from build123d import *

# Parameters (mm, degrees)
BOSS_EXTRUDE1_DEPTH      = 19.05
BOSS_EXTRUDE1_DEPTH_BACK = 54.61
SKETCH2_R                = 3.2512
CUT_EXTRUDE1_DEPTH       = 9.525
FILLET1_R                = 1.27


with BuildPart() as part:
    # Sketch1 → Boss-Extrude1 (new, two sides: drawn at the far end of the back side and taken through both)
    with BuildSketch(Plane(origin=(0, 0, 0), x_dir=(1, 0, 0), z_dir=(0, 1, 0)).offset(-BOSS_EXTRUDE1_DEPTH_BACK)):
        with BuildLine():
            Line((6.1595, -12.990051451), (6.1595, -27.747157521))
            ThreePointArc((6.1595, -27.747157521), (0, -28.4226), (-6.1595, -27.747157521))
            Line((-6.1595, -27.747157521), (-6.1595, -12.990051451))
            ThreePointArc((-6.1595, -12.990051451), (0, -14.3764), (6.1595, -12.990051451))
        make_face()
    extrude(amount=BOSS_EXTRUDE1_DEPTH + BOSS_EXTRUDE1_DEPTH_BACK)

    # Sketch2 → Cut-Extrude1 (cut, symmetric)
    with BuildSketch(Plane(origin=(0, 0, 0), x_dir=(0, 0, -1), z_dir=(1, 0, 0))):
        with Locations((-20.6375, 12.7)):
            Circle(SKETCH2_R)
        with Locations((-20.6375, -48.26)):
            Circle(SKETCH2_R)
    extrude(amount=CUT_EXTRUDE1_DEPTH, both=True, mode=Mode.SUBTRACT)

    # Fillet1
    fillet1_edges = [part.edges().sort_by_distance(p)[0] for p in [
        (0, -54.61, 28.4226),
        (0, 19.05, 14.3764),
        (-6.1595, 19.05, 20.368604486),
        (6.1595, -54.61, 20.368604486),
        (0, 19.05, 28.4226),
        (6.1595, 19.05, 20.368604486),
        (0, -54.61, 14.3764),
        (-6.1595, -54.61, 20.368604486),
        (6.1595, -17.78, 12.990051451),
        (6.1595, -17.78, 27.747157521),
        (-6.1595, -17.78, 27.747157521),
        (-6.1595, -17.78, 12.990051451),
    ]]
    fillet(fillet1_edges, radius=FILLET1_R)


solid = part.part
Read the model definition and answer for the solid it produces. Units are mm, in the model's axes. Coordinates: 2 decimals unless noted, no trailing zeros. Order: outer loops, then holes, each group sorted by start corner. A loop starts at its lowest first (then second) coordinate and runs counter-clockwise, first axis right, second up. Notation, with made-up numbers: (17, 74) - (29, 74) arc R20 ccw to (29, 98) - close; hole circle Ø10 at (-26.5, 53). An arc over 180 degrees is marked (long way). Use one line per item in the form item = value.
(1) Given pin 1 Ø4 at (x, y) = (0.5, -25) entering from -Z; pin 2 Ø6 at (x, y) = (3.5, -17) entering from +Z; pin 3 Ø1.5 at (x, y) = (3.5, -14.5) entering from -Z, each flat-ended and moving along its own axis, determine where each tip first touches the part or whether it passes through.
Computed values:
pin_1 = 14.16
pin_2 = 28.42
pin_3 = 13.73
(2) Section D-D, the plane z = 18.5 is taken. Give the vertices of the cut face in (x, y).
Computed values:
outline = (-6.16, -53.34) arc R1.27 ccw to (-4.89, -54.61) - (4.89, -54.61) arc R1.27 ccw to (6.16, -53.34) - (6.16, -50.71) - (-6.16, -50.71) - close; (-6.16, -45.81) - (6.16, -45.81) - (6.16, 10.25) - (-6.16, 10.25) - close; (-6.16, 15.15) - (6.16, 15.15) - (6.16, 17.78) arc R1.27 ccw to (4.89, 19.05) - (-4.89, 19.05) arc R1.27 ccw to (-6.16, 17.78) - close
(3) Section A-A, the plane y = 12.7 is taken. Give the vertices of the cut face in (x, z), then the cut area to 3 significant figures.
Computed values:
outline = (-6.16, 14.86) arc R1.27 ccw to (-4.49, 13.66) arc R14.38 cw to (4.49, 13.66) arc R1.27 ccw to (6.16, 14.86) - (6.16, 17.39) - (-6.16, 17.39) - close; (-6.16, 23.89) - (6.16, 23.89) - (6.16, 26.71) arc R1.27 ccw to (5.12, 27.96) arc R28.42 ccw to (-5.12, 27.96) arc R1.27 ccw to (-6.16, 26.71) - close
area = 93.8 mm²
(4) Section B-B, the plane z = 22 is taken. Give the vertices of the cut face in (x, y), then the cut area to 3 significant figures.
Computed values:
outline = (-6.16, -53.34) arc R1.27 ccw to (-4.89, -54.61) - (4.89, -54.61) arc R1.27 ccw to (6.16, -53.34) - (6.16, -51.21) - (-6.16, -51.21) - close; (-6.16, -45.31) - (6.16, -45.31) - (6.16, 9.75) - (-6.16, 9.75) - close; (-6.16, 15.65) - (6.16, 15.65) - (6.16, 17.78) arc R1.27 ccw to (4.89, 19.05) - (-4.89, 19.05) arc R1.27 ccw to (-6.16, 17.78) - close
area = 761 mm²
(5) For a pull along Z with two mould halves and no side action, classify faces 1 (the face through (-6.16, -18, 21)), 2 (the face through (0.072, -18.278, 28.423)), 3 (the face through (0.086, -51.144, 19.137)) as pulls with the +Z half, pulls with the -Z half, needs draft (parallel to the pull), parting line crosses it, or undercut.
Computed values:
face_1 = needs draft
face_2 = pulls with the +Z half
face_3 = undercut
(6) Straight lines are drawn through the part: L1, parallel to Y at x = 0.75, z = 20.5; L2, parallel to Y at x = 5, z = 19.5; L3, parallel to Z at x = 3.5, y = 12.7. For each, find the intervals that lie inside material, in ascending order.
Computed values:
L1 = -54.61 to -51.51, -45.01 to 9.45, 15.95 to 19.05
L2 = -54.61 to -51.31, -45.21 to 9.65, 15.75 to 19.05
L3 = 13.94 to 17.39, 23.89 to 28.21
(7) Section C-C, the plane y = 0 is taken. Give the vertices of the cut face in (x, z), then the cut area to 3 significant figures.
Computed values:
outline = (-6.16, 14.86) arc R1.27 ccw to (-4.49, 13.66) arc R14.38 cw to (4.49, 13.66) arc R1.27 ccw to (6.16, 14.86) - (6.16, 26.71) arc R1.27 ccw to (5.12, 27.96) arc R28.42 ccw to (-5.12, 27.96) arc R1.27 ccw to (-6.16, 26.71) - close
area = 174 mm²
